```python
from build123d import *

# Parameters (mm, degrees)
CUT_EXTRUDE_START       = -6
CUT_EXTRUDE_4_OUTLINE_R = 6.5
CUT_EXTRUDE_4_DEPTH     = 6
SKETCH_1_6_R            = 6.65
CUT_EXTRUDE_5_DEPTH     = 10
SKETCH_1_7_W            = 120.462330866
SKETCH_1_7_H            = 12.505444566
EXTRUDE_1_DEPTH         = 6
CUT_EXTRUDE_6_DEPTH     = 6
EXTRUDE_START           = -6
SKETCH_3_R              = 6.65
EXTRUDE_3_DEPTH         = 6


with BuildPart() as part:
    # 切除-拉伸4: read off the stored shape, not the designer's step
    # 切除-拉伸4 outline → 切除-拉伸4 (new body)
    with BuildSketch(Plane.ZY.offset(3).offset(CUT_EXTRUDE_START)):
        with BuildLine():
            Line((-160, -12), (-16.278820596, -12))
            ThreePointArc((-16.278820596, -12), (-12.755499279, -12.528896875), (-9.542756901, -14.068965517))
            ThreePointArc((-9.542756901, -14.068965517), (17, 0), (-9.542756901, 14.068965517))
            ThreePointArc((-9.542756901, 14.068965517), (-12.755499279, 12.528896875), (-16.278820596, 12))
            Line((-16.278820596, 12), (-160, 12))
            ThreePointArc((-160, 12), (-172, 0), (-160, -12))
        make_face()
        with Locations((-160, 0)):
            Circle(CUT_EXTRUDE_4_OUTLINE_R, mode=Mode.SUBTRACT)
        with BuildLine():
            Line((-120, -3), (-134, -3))
            ThreePointArc((-134, -3), (-137, 0), (-134, 3))
            Line((-134, 3), (-120, 3))
            ThreePointArc((-120, 3), (-117, 0), (-120, -3))
        make_face(mode=Mode.SUBTRACT)
        with BuildLine():
            Line((-90, -3), (-104, -3))
            ThreePointArc((-104, -3), (-107, 0), (-104, 3))
            Line((-104, 3), (-90, 3))
            ThreePointArc((-90, 3), (-87, 0), (-90, -3))
        make_face(mode=Mode.SUBTRACT)
        with BuildLine():
            Line((-60, -3), (-74, -3))
            ThreePointArc((-74, -3), (-77, 0), (-74, 3))
            Line((-74, 3), (-60, 3))
            ThreePointArc((-60, 3), (-57, 0), (-60, -3))
        make_face(mode=Mode.SUBTRACT)
        with BuildLine():
            Line((-30, -3), (-44, -3))
            ThreePointArc((-44, -3), (-47, 0), (-44, 3))
            Line((-44, 3), (-30, 3))
            ThreePointArc((-30, 3), (-27, 0), (-30, -3))
        make_face(mode=Mode.SUBTRACT)
        with BuildLine():
            ThreePointArc((-5.4816883, -4.494562647), (-5.376440838, -4.232531174), (-5.348640266, -3.951524681))
            ThreePointArc((-5.348640266, -3.951524681), (-6.65, 0), (-5.348640266, 3.951524681))
            ThreePointArc((-5.348640266, 3.951524681), (-5.376440838, 4.232531174), (-5.4816883, 4.494562647))
            Line((-5.4816883, 4.494562647), (-6.100603614, 5.566555416))
            ThreePointArc((-6.100603614, 5.566555416), (-5.7, 9.872689603), (-1.770476595, 8.066555416))
            Line((-1.770476595, 8.066555416), (-1.151561281, 6.994562647))
            ThreePointArc((-1.151561281, 6.994562647), (-0.9772591, 6.772399934), (-0.747800624, 6.607820687))
            ThreePointArc((-0.747800624, 6.607820687), (3.325, 5.759068935), (6.09644089, 2.656296006))
            ThreePointArc((6.09644089, 2.656296006), (6.353699938, 2.53986876), (6.633249581, 2.5))
            Line((6.633249581, 2.5), (7.871080208, 2.5))
            ThreePointArc((7.871080208, 2.5), (11.4, 0), (7.871080208, -2.5))
            Line((7.871080208, -2.5), (6.633249581, -2.5))
            ThreePointArc((6.633249581, -2.5), (6.353699938, -2.53986876), (6.09644089, -2.656296006))
            ThreePointArc((6.09644089, -2.656296006), (3.325, -5.759068935), (-0.747800624, -6.607820687))
            ThreePointArc((-0.747800624, -6.607820687), (-0.9772591, -6.772399934), (-1.151561281, -6.994562647))
            Line((-1.151561281, -6.994562647), (-1.770476595, -8.066555416))
            ThreePointArc((-1.770476595, -8.066555416), (-5.7, -9.872689603), (-6.100603614, -5.566555416))
            Line((-6.100603614, -5.566555416), (-5.4816883, -4.494562647))
        make_face(mode=Mode.SUBTRACT)
    extrude(amount=CUT_EXTRUDE_4_DEPTH)

    # 草图1<6> → 切除-拉伸5 (cut)
    with BuildSketch(Plane.ZY.offset(3)):
        with Locations((-160, 0)):
            Circle(SKETCH_1_6_R)
    extrude(amount=-CUT_EXTRUDE_5_DEPTH, mode=Mode.SUBTRACT)

    # 草图1<7> → 凸台-拉伸1 (add)
    with BuildSketch(Plane.ZY.offset(3)):
        with Locations((-81.625615337, 0)):
            Rectangle(SKETCH_1_7_W, SKETCH_1_7_H)
    extrude(amount=-EXTRUDE_1_DEPTH)

    # 草图2 → 切除-拉伸6 (cut)
    with BuildSketch(Plane.ZY.offset(3)):
        with BuildLine():
            Line((-130, 3), (-110, 3))
            ThreePointArc((-110, 3), (-107, 0), (-110, -3))
            Line((-110, -3), (-130, -3))
            ThreePointArc((-130, -3), (-133, 0), (-130, 3))
        make_face()
        with BuildLine():
            Line((-90, 3), (-70, 3))
            ThreePointArc((-70, 3), (-67, 0), (-70, -3))
            Line((-70, -3), (-90, -3))
            ThreePointArc((-90, -3), (-93, 0), (-90, 3))
        make_face()
        with BuildLine():
            Line((-50, 3), (-30, 3))
            ThreePointArc((-30, 3), (-27, 0), (-30, -3))
            Line((-30, -3), (-50, -3))
            ThreePointArc((-50, -3), (-53, 0), (-50, 3))
        make_face()
    extrude(amount=-CUT_EXTRUDE_6_DEPTH, mode=Mode.SUBTRACT)

    # 草图3 → 凸台-拉伸3 (add)
    # profile 1 of 6: a face of its own
    with BuildSketch(Plane.ZY.offset(3).offset(EXTRUDE_START)):
        with BuildLine():
            Line((0, 17), (-160, 17))
            ThreePointArc((-160, 17), (-153.480797595, 15.700318468), (-147.958405421, 12))
            Line((-147.958405421, 12), (-16.278820596, 12))
            ThreePointArc((-16.278820596, 12), (-12.755499279, 12.528896875), (-9.542756901, 14.068965517))
            ThreePointArc((-9.542756901, 14.068965517), (-4.991371866, 16.250729427), (0, 17))
        make_face()
    # profile 2 of 6: a face of its own
    with BuildSketch(Plane.ZY.offset(3).offset(EXTRUDE_START)):
        with BuildLine():
            Line((-16.278820596, 12), (-147.958405421, 12))
            ThreePointArc((-147.958405421, 12), (-146.052319534, 9.719167126), (-144.57264474, 7.141198057))
            Line((-144.57264474, 7.141198057), (-15.42735526, 7.141198057))
            ThreePointArc((-15.42735526, 7.141198057), (-12.95666299, 11.005675089), (-9.542756901, 14.068965517))
            ThreePointArc((-9.542756901, 14.068965517), (-12.755499279, 12.528896875), (-16.278820596, 12))
        make_face()
    # profile 3 of 6: a face of its own
    with BuildSketch(Plane.ZY.offset(3).offset(EXTRUDE_START)):
        with BuildLine():
            ThreePointArc((-143.664552767, -4.706714744), (-145.350353999, -8.624840407), (-147.958405421, -12))
            Line((-147.958405421, -12), (-16.278820596, -12))
            ThreePointArc((-16.278820596, -12), (-12.755499279, -12.528896875), (-9.542756901, -14.068965517))
            ThreePointArc((-9.542756901, -14.068965517), (-13.759843647, -9.983321231), (-16.335447233, -4.706714744))
            Line((-16.335447233, -4.706714744), (-143.664552767, -4.706714744))
        make_face()
    # profile 4 of 6: a face of its own
    with BuildSketch(Plane.ZY.offset(3).offset(EXTRUDE_START)):
        with BuildLine():
            ThreePointArc((-147.958405421, -12), (-153.480797595, -15.700318468), (-160, -17))
            Line((-160, -17), (0, -17))
            ThreePointArc((0, -17), (-4.991371866, -16.250729427), (-9.542756901, -14.068965517))
            ThreePointArc((-9.542756901, -14.068965517), (-12.755499279, -12.528896875), (-16.278820596, -12))
            Line((-16.278820596, -12), (-147.958405421, -12))
        make_face()
    # profile 5 of 6: a face of its own
    with BuildSketch(Plane.ZY.offset(3).offset(EXTRUDE_START)):
        with BuildLine():
            ThreePointArc((-144.57264474, 7.141198057), (-146.052319534, 9.719167126), (-147.958405421, 12))
            Line((-147.958405421, 12), (-160, 12))
            ThreePointArc((-160, 12), (-172, 0), (-160, -12))
            Line((-160, -12), (-147.958405421, -12))
            ThreePointArc((-147.958405421, -12), (-145.350353999, -8.624840407), (-143.664552767, -4.706714744))
            ThreePointArc((-143.664552767, -4.706714744), (-143.166958044, -2.37669908), (-143, 0))
            ThreePointArc((-143, 0), (-143.397815815, 3.656156492), (-144.57264474, 7.141198057))
        make_face()
        with Locations((-160, 0)):
            Circle(SKETCH_3_R, mode=Mode.SUBTRACT)
    # profile 6 of 6: a face of its own
    with BuildSketch(Plane.ZY.offset(3).offset(EXTRUDE_START)):
        with BuildLine():
            ThreePointArc((-147.958405421, 12), (-153.480797595, 15.700318468), (-160, 17))
            ThreePointArc((-160, 17), (-177, 0), (-160, -17))
            ThreePointArc((-160, -17), (-153.480797595, -15.700318468), (-147.958405421, -12))
            Line((-147.958405421, -12), (-160, -12))
            ThreePointArc((-160, -12), (-172, 0), (-160, 12))
            Line((-160, 12), (-147.958405421, 12))
        make_face()
    extrude(amount=EXTRUDE_3_DEPTH)


solid = part.part
```
Work out the finished part from the listing and answer in its coordinate system (mm). A direction names the side the tool comes from. Give positions to 0.01 mm unless a question says otherwise; leave off trailing zeros. Loops run counter-clockwise (first coordinate to the right, second up) from the corner with the lowest first, then second, coordinate; pieces in that order, holes last. Notation, with made-up numbers: M -4,56 L 13,56 A36 ccw 13,93 Z; hole C -19.75,46 d6. An arc over 180 degrees is marked long. One line per item, written item: value. Start each with the question number.
1. Which of the six approach directions +Z, -Z, +X, -X, +Y, -Y give full straight-line access (tool end or side, diameter ignored) to faces 4 (the face through (0, 17, -79)), 5 (the face through (0, 0, -53))?
2. Find the intervals of material crossed by probe 1 along Z at (x, y) = (2.35, -5.5); probe 2 along Y at (x, z) = (-0.1, -42); probe 3 along Y at (x, z) = (-1.4, -160), in increasing order.
3. Find section A-A (z = -32). Give the vertices of the cut face in (x, y), and give its area (3 significant figures).
4. Each of these flat-tipped pins is pushed along its axis until it touches: P1, Ø3, axis at y = 7.58, z = -4.38, coming from the -X side; P2, Ø3, axis at x = 0, y = -7.5, coming from the -Z side; P3, Ø1, axis at x = -0.5, z = 7.5, coming from the -Y side; P4, Ø0.6, axis at x = -1, z = 7, coming from the +Y side. Where does it stop, or does it pass through?
5. Find section B-B (x = -1.1). State how many separate pieces and enclosed holes the cut face has, and give its area (3 significant figures).
6. Find section C-C (y = 12.5). Give the vertices of the cut face in (x, z).
7. Determine the mould class of faces 1 (the face through (0, 0, -67)), 2 (the face through (-3, -4, -81)), 3 (the face through (0, 0, 17)) for opening direction Y: released by +Y, released by -Y, zero draft, split by the parting line, or undercut.
Reported:
1. face 4: +Z, -Z, +X, -X, +Y
1. face 5: +X, -X
2. probe 1: z = -176.09 to -163.74, -156.26 to -6.06, 3.74 to 16.09
2. probe 2: y = -17 to -3, 3 to 17
2. probe 3: y = -17 to -6.65, 6.65 to 17
3. outline: M -3,-17 L 3,-17 L 3,-3 L -3,-3 Z; M -3,3 L 3,3 L 3,17 L -3,17 Z
3. area: 168 mm²
4. P1: passes through
4. P2: stops at z = -175.91
4. P3: stops at y = -15.49
4. P4: stops at y = 15.62
5. separate pieces: 1
5. enclosed holes: 5
5. area: 5,560 mm²
6. outline: M -3,-171.52 L 3,-171.52 L 3,11.52 L -3,11.52 Z
7. face 1: undercut
7. face 2: zero draft
7. face 3: split by the parting line
